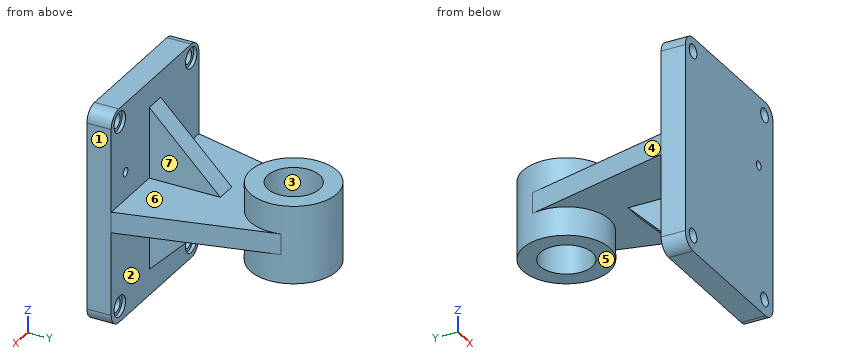
```python
from build123d import *

# Parameters (mm, degrees)
SKETCH_1_R                   = 25
SKETCH_1_R_2                 = 15
EXTRUDE_1_DEPTH              = 22.5
SKETCH_2_W                   = 92
SKETCH_2_H                   = 14
EXTRUDE_2_DEPTH              = 62
EXTRUDE_3_DEPTH              = 6
RIB_1_REACH                  = 123.639
SKETCH_4_WALL_W              = 303.26037525
SKETCH_4_WALL_H              = 12
FILLET_1_R                   = 8
HOLE_WIZARD_M5_1_D           = 8
HOLE_WIZARD_M5_1_CBORE_D     = 12
HOLE_WIZARD_M5_1_CBORE_DEPTH = 2
HOLE_WIZARD_M6_1_D           = 5
PATTERN_LINEAR_7_COUNT       = 2
PATTERN_LINEAR_7_PITCH       = 75
PATTERN_LINEAR_7_COUNT_DIR2  = 2
PATTERN_LINEAR_7_PITCH_DIR2  = 107


with BuildPart() as part:
    # Sketch 1 → Extrude 1 (new, symmetric)
    with BuildSketch(Plane.XY):
        with Locations(Location((0, 0, 0), (0, 0, 180))):
            Circle(SKETCH_1_R)
        with Locations(Location((0, 0, 0), (0, 0, 180))):
            Circle(SKETCH_1_R_2, mode=Mode.SUBTRACT)
    extrude(amount=EXTRUDE_1_DEPTH, both=True)



with BuildPart() as body_2:
    # Sketch 2 → Extrude 2 (new, symmetric)
    with BuildSketch(Plane.XY):
        with Locations((0, -87)):
            Rectangle(SKETCH_2_W, SKETCH_2_H)
    extrude(amount=EXTRUDE_2_DEPTH, both=True)


with BuildPart() as part_1:
    add(part.part)

    add(body_2.part)  # Extrude 3 merges body 2
    # Sketch 3 → Extrude 3 (add, symmetric)
    with BuildSketch(Plane.XY):
        with BuildLine():
            Line((-24.238210613, 6.124471102), (-46, -80))
            Line((-46, -80), (46, -80))
            Line((46, -80), (24.238210613, 6.124471102))
            ThreePointArc((24.238210613, 6.124471102), (0, -25), (-24.238210613, 6.124471102))
        make_face()
    extrude(amount=EXTRUDE_3_DEPTH, both=True)

    # Sketch 4 wall → Rib 1 (add, up to next)
    with BuildSketch(Plane(origin=(0, -59.5, 26.5), x_dir=(0, -0.707106781187, 0.707106781187), z_dir=(0, -0.707106781187, -0.707106781187)), mode=Mode.PRIVATE) as rib_1_sk1:
        Rectangle(SKETCH_4_WALL_W, SKETCH_4_WALL_H)
    rib_1_tool1 = extrude(rib_1_sk1.sketch, amount=RIB_1_REACH, mode=Mode.PRIVATE) - part_1.part
    rib_1 = rib_1_tool1.solids().sort_by_distance((0, -59.5, 26.5))[0]
    add(rib_1)

    # Mirror 1: Rib 1 across plane
    add(rib_1.mirror(Plane.XY))

    # Fillet 1
    fillet_1_edges = [part_1.edges().sort_by_distance(p)[0] for p in [
        (-46, -87, -62),
        (46, -87, 62),
        (46, -87, -62),
        (-46, -87, 62),
    ]]
    fillet(fillet_1_edges, radius=FILLET_1_R)

    # Hole Wizard M5 _ _ _ _ _1 (through all)
    with Locations(Plane(origin=(-38, -80, 54), x_dir=(0, 0, 1), z_dir=(0, 1, 0))):
        with Locations((0, 0)):
            hole_wizard_m5_1 = CounterBoreHole(HOLE_WIZARD_M5_1_D / 2, HOLE_WIZARD_M5_1_CBORE_D / 2, HOLE_WIZARD_M5_1_CBORE_DEPTH)

    # Hole Wizard M6 _ _1 (through all)
    with Locations(Plane(origin=(30.943238256, -80, 21.843950173), x_dir=(0, 0, 1), z_dir=(0, 1, 0))):
        with Locations((0, 0)):
            Hole(HOLE_WIZARD_M6_1_D / 2)

    # Pattern Linear 7: Hole Wizard M5 _ _ _ _ _1 2 × 2
    with Locations(*[(i * PATTERN_LINEAR_7_PITCH, 0, -j * PATTERN_LINEAR_7_PITCH_DIR2) for i in range(PATTERN_LINEAR_7_COUNT) for j in range(PATTERN_LINEAR_7_COUNT_DIR2) if (i, j) != (0, 0)]):
        add(hole_wizard_m5_1, mode=Mode.SUBTRACT)


solid = part_1.part
```
Source: CAD feature listing. Evaluate the final solid. Frame: model axes, mm. Face numbers are marked on the shaded views. A direction names the side the tool comes from. Give positions to 0.01 mm unless a question says otherwise; leave off trailing zeros. Write each loop counter-clockwise with the first axis right and the second up, starting at its lowest first coordinate (ties: lowest second). Pieces come first, ordered by that corner, then holes. Notation, with made-up numbers: (-33, 62.5) - (-11, 62.5) arc R22 ccw to (-11, 80.5) - close; hole circle Ø8 at (50, 58). An arc over 180 degrees is marked (long way). One line per item, written item: value. Start each with the question number.
Q1. Section query B-B, the plane y = -5. Return the cut outline in (x, z).
Q2. Section query C-C, the plane y = 9.5. Return the cut outline in (x, z), then the cut area to 3 significant figures.
Q3. Material intervals for probe 1 along X at (y, z) = (-80.9, 54); probe 2 along Y at (x, z) = (-20, 14.5); probe 3 along Z at (x, y) = (-9, -38), sorted ascending. Write a range as from..to.
Q4. Draft query along Y for the marked faces 1, 2, 3 and 4. Return one class per face: +Y half, -Y half, draft (parallel to the pull), parting line (faces both ways), or undercut.
Q5. First-contact query: pin 1 Ø13 at (x, z) = (37, -53) entering from +Y; pin 2 Ø6 at (x, z) = (-37.5, 53) entering from +Y; pin 3 Ø1 at (x, y) = (9.5, -46) entering from +Z. Flat tips, straight axial feed; report the tip coordinate or a pass-through.
Q6. Section query A-A, the plane x = 0. Return the cut outline in (y, z).
Q7. Set-up query: the marked faces 5, 6 and 7. Return all of +Z, -Z, +X, -X, +Y, -Y with unobstructed straight access to the full face (end or side cutting, diameter ignored); none if empty.
Answer:
1. outline: (-27.05, -6) - (-24.49, -6) - (-24.49, -22.5) - (-14.14, -22.5) - (-14.14, 22.5) - (-24.49, 22.5) - (-24.49, 6) - (-27.05, 6) - close; (14.14, -22.5) - (24.49, -22.5) - (24.49, -6) - (27.05, -6) - (27.05, 6) - (24.49, 6) - (24.49, 22.5) - (14.14, 22.5) - close
2. outline: (-23.12, -22.5) - (-11.61, -22.5) - (-11.61, 22.5) - (-23.12, 22.5) - close; (11.61, -22.5) - (23.12, -22.5) - (23.12, 22.5) - (11.61, 22.5) - close
2. area: 1,040 mm2
3. probe 1: x = -46..-44, -32..31, 43..46
3. probe 2: y = -94..-80, -15..15
3. probe 3: z = -6..6
4. face 1: draft
4. face 2: undercut
4. face 3: undercut
4. face 4: +Y half
5. pin 1: stops at y = -80
5. pin 2: stops at y = -82
5. pin 3: stops at z = 6
6. outline: (-94, -62) - (-80, -62) - (-80, -47) - (-39, -6) - (-25, -6) - (-25, -22.5) - (-15, -22.5) - (-15, 22.5) - (-25, 22.5) - (-25, 6) - (-39, 6) - (-80, 47) - (-80, 62) - (-94, 62) - close; (15, -22.5) - (25, -22.5) - (25, 22.5) - (15, 22.5) - close
7. face 5: -Z, +X, -X, +Y
7. face 6: +Z
7. face 7: +Z, +X
